Could you check a few things on this model? Use its own coordinates, in mm. Face numbers are marked on the shaded views. Give positions to 0.01 mm unless a question says otherwise; leave off trailing zeros. Loops run counter-clockwise (first coordinate to the right, second up) from the corner with the lowest first, then second, coordinate; pieces in that order, holes last. Notation, with made-up numbers: (-37.5, -11) - (8.5, -11) arc R18 ccw to (8.5, 20) - close; hole circle Ø8 at (-14, -32). An arc over 180 degrees is marked (long way). Write each question's results on one line, items separated by ' | '. Start each with the question number.
1) I'm going to push flat-ended pins straight in: pin 1 (3 mm diameter, centred on x = -2.5, z = -0.5, fed in from -Y); pin 2 (1 mm diameter, centred on x = 1.5, y = 12, fed in from +Z); pin 3 (1.6 mm diameter, centred on x = 2, y = 12.5, fed in from -Z). Where does each tip first touch, or does it pass through?
2) If I drill on probe 1 along Y at (x, z) = (-1.25, 0); probe 2 along Z at (x, y) = (2.5, 12.5); probe 3 along Y at (x, z) = (-2.5, 27), over which ranges is the centre line in solid material (lowest first)? Write a range as [from, to].
3) I want a section at C-C, the plane x = -3.25. Write out the boundary of the cut face in (y, z).
4) I want a section at D-D, the plane y = -53. Write out the boundary of the cut face in (x, z).
5) I want a section at A-A, the plane z = 0. Write out the boundary of the cut face in (x, y), and give its area (3 significant figures).
6) If we mould it in two halves opening along Z, with no side actions, what happens to the marked faces 1, 2 and 3? For each: +Z half, -Z half, draft (parallel to the pull), parting line (faces both ways), or undercut.
7) I want a section at B-B, the plane y = 0. Write out the boundary of the cut face in (x, z).
from build123d import *

# Parameters (mm, degrees)
SKETCH1_R           = 65
BOSS_EXTRUDE1_DEPTH = 5
SKETCH3_R           = 11
CUT_EXTRUDE2_DEPTH  = 93.466210045
CUT_EXTRUDE5_DEPTH  = 93.466210045


with BuildPart() as part:
    # Sketch1 → Boss-Extrude1 (new, symmetric)
    with BuildSketch(Plane(origin=(0, 0, 0), x_dir=(0, 0, -1), z_dir=(1, 0, 0))):
        Circle(SKETCH1_R)
    extrude(amount=BOSS_EXTRUDE1_DEPTH, both=True)

    # Sketch3 → Cut-Extrude2 (cut, through all)
    with BuildSketch(Plane(origin=(5, 0, 0), x_dir=(0, 0, -1), z_dir=(1, 0, 0))):
        Circle(SKETCH3_R)
    extrude(amount=-CUT_EXTRUDE2_DEPTH, mode=Mode.SUBTRACT)

    # Sketch5 → Cut-Extrude5 (cut, through all)
    with BuildSketch(Plane(origin=(5, 0, 0), x_dir=(0, 0, -1), z_dir=(1, 0, 0))):
        with BuildLine():
            Line((-2, 10.816653826), (-2, 12.816653826))
            Line((-2, 12.816653826), (2, 12.816653826))
            Line((2, 12.816653826), (2, 10.816653826))
            ThreePointArc((2, 10.816653826), (0, 11), (-2, 10.816653826))
        make_face()
    extrude(amount=-CUT_EXTRUDE5_DEPTH, mode=Mode.SUBTRACT)


solid = part.part
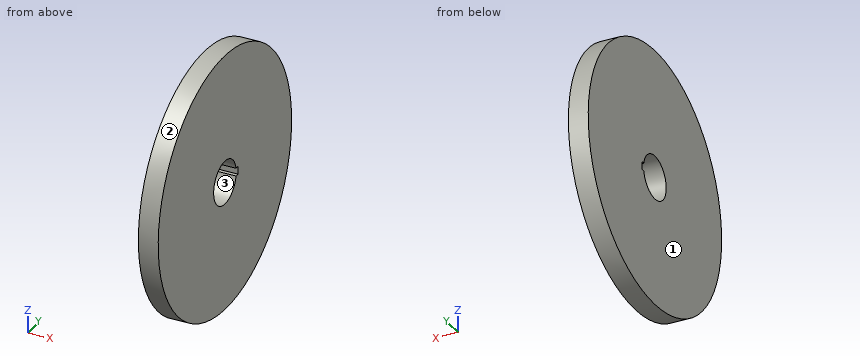
Answers:
1) pin 1: stops at y = -65 | pin 2: stops at z = 63.97 | pin 3: stops at z = -63.94
2) probe 1: y = [-65, -11], [12.82, 65] | probe 2: z = [-63.79, -2], [2, 63.79] | probe 3: y = [-59.13, 59.13]
3) outline: circle Ø130 at (0, 0); hole (10.82, -2) - (12.82, -2) - (12.82, 2) - (10.82, 2) arc R11 ccw (long way) to start
4) outline: (-5, -37.63) - (5, -37.63) - (5, 37.63) - (-5, 37.63) - close
5) outline: (-5, -65) - (5, -65) - (5, -11) - (-5, -11) - close; (-5, 12.82) - (5, 12.82) - (5, 65) - (-5, 65) - close | area: 1,060 mm2
6) face 1: draft | face 2: parting line | face 3: undercut
7) outline: (-5, -65) - (5, -65) - (5, -11) - (-5, -11) - close; (-5, 11) - (5, 11) - (5, 65) - (-5, 65) - close
